from build123d import *

# Parameters (mm, degrees)
F1_DEPTH = 4.5
F2_DEPTH = 4.501
F3_DEPTH = 1
F4_R     = 2


# Not quite as in the source:
# - a feature names something its author has since deleted; it is built from what else it names


with BuildPart() as f1:
    # F0 (on Front) → F1 (new body)
    with BuildSketch(Plane.XZ):
        Polygon((25, 12.5), (-25, 12.5), (-25, 4), (-25, -4), (-25, -12.5), (25, -12.5), (25, -4), (25, 4), align=None)
        Polygon((-23.25, 7.75), (-23.25, 10.75), (-20.25, 10.75), (20.25, 10.75), (23.25, 10.75), (23.25, 7.75), (23.25, -7.75), (23.25, -10.75), (20.25, -10.75), (-20.25, -10.75), (-23.25, -10.75), (-23.25, -7.75), align=None, mode=Mode.SUBTRACT)
        Polygon((-20.25, 10.75), (-23.25, 10.75), (-23.25, 7.75), align=None)
        Polygon((23.25, 10.75), (20.25, 10.75), (23.25, 7.75), align=None)
        with BuildLine():
            Line((-25, -4), (-25, 4))
            Line((-25, 4), (-29.5, 4))
            ThreePointArc((-29.5, 4), (-33.5, 0), (-29.5, -4))
            Line((-29.5, -4), (-25, -4))
        make_face()
        with BuildLine():
            Line((-28.5, -1.8), (-29.5, -1.8))
            ThreePointArc((-29.5, -1.8), (-31.3, 0), (-29.5, 1.8))
            Line((-29.5, 1.8), (-28.5, 1.8))
            ThreePointArc((-28.5, 1.8), (-26.7, 0), (-28.5, -1.8))
        make_face(mode=Mode.SUBTRACT)
        with BuildLine():
            Line((29.5, 4), (25, 4))
            Line((25, 4), (25, -4))
            Line((25, -4), (29.5, -4))
            ThreePointArc((29.5, -4), (33.5, 0), (29.5, 4))
        make_face()
        with BuildLine():
            ThreePointArc((29.5, 1.8), (31.3, 0), (29.5, -1.8))
            Line((29.5, -1.8), (28.5, -1.8))
            ThreePointArc((28.5, -1.8), (26.7, 0), (28.5, 1.8))
            Line((28.5, 1.8), (29.5, 1.8))
        make_face(mode=Mode.SUBTRACT)
    extrude(amount=F1_DEPTH)

    # F0 (on Front) → F2 (cut, through all)
    with BuildSketch(Plane.XZ):
        Polygon((-20.25, 10.75), (-23.25, 10.75), (-23.25, 7.75), align=None)
        Polygon((20.25, 10.75), (-20.25, 10.75), (-23.25, 7.75), (-23.25, -7.75), (-20.25, -10.75), (20.25, -10.75), (23.25, -7.75), (23.25, 7.75), align=None)
        Polygon((23.25, 10.75), (20.25, 10.75), (23.25, 7.75), align=None)
    extrude(amount=F2_DEPTH, mode=Mode.SUBTRACT)

    # F0 (on Front) → F3 (join)
    with BuildSketch(Plane.XZ):
        Polygon((23.25, 10.75), (20.25, 10.75), (23.25, 7.75), align=None)
        Polygon((23.25, -10.75), (23.25, -7.75), (20.25, -10.75), align=None)
        Polygon((-20.25, 10.75), (-23.25, 10.75), (-23.25, 7.75), align=None)
        Polygon((-20.25, -10.75), (-23.25, -7.75), (-23.25, -10.75), align=None)
    extrude(amount=F3_DEPTH)

    # F4
    f4_edges = [f1.edges().sort_by_distance(p)[0] for p in [
        (-25, -2.25, -12.5),
        (25, -2.25, -12.5),
        (25, -2.25, 12.5),
        (-25, -2.25, 12.5),
    ]]
    fillet(f4_edges, radius=F4_R)


solid = f1.part
Source: CAD feature listing. Evaluate the final solid. Frame: model axes, mm. A direction names the side the tool comes from. Round coordinates to 2 decimals unless told otherwise and drop trailing zeros. Loops run counter-clockwise (first coordinate to the right, second up) from the corner with the lowest first, then second, coordinate; pieces in that order, holes last. Notation, with made-up numbers: M 23,60 L 41,60 A32 ccw 41,99 Z; hole C 50.25,-40 d1. An arc over 180 degrees is marked long. Return JSON: item names as keys, results as strings. Group by question number.
1. Reachability of faces 1 (the face through (-27, -2, 4)), 2 (the face through (-21.8, -0.5, 9.2)), 3 (the face through (22, -1, -10)) from +Z, -Z, +X, -X, +Y, -Y: full face, straight path, thin tool, end or side. Return the list, or none.
2. Mould query, pull axis Z, two halves, no side actions, for faces 4 (the face through (-21.7, -0.5, -9.3)), 5 (the face through (27, -2, 4)), 6 (the face through (24.4, -2.28, -11.93)), 7 (the face through (-25, -2, -7)). Classes: released by +Z, released by -Z, zero draft, split by the parting line, or undercut.
3. Section query A-A on x = -9. Output: boundary loops of the cut face in (y, z), and give its area (4 significant figures).
4. Section query C-C on y = -1.85. Output: boundary loops of the cut face in (x, z), and give its area (3 significant figures).
5. Section query B-B on z = 6.5. Output: boundary loops of the cut face in (x, y), and give its area (4 significant figures).
6. Material intervals for line 1 along Z through (x, y) = (-9.5, -3); line 2 along X through (y, z) = (-4.05, -4.25); line 3 along X through (y, z) = (-0.8, -8), sorted ascending. Write a range as from..to.
7. Pin query (flat end, axial travel): pin 1 (2 mm diameter, centred on x = 27, y = -1.5, fed in from +Z); pin 2 (2 mm diameter, centred on y = -1.5, z = -7, fed in from -X); pin 3 (1.5 mm diameter, centred on x = 22, z = -9, fed in from -Y). Return the tip coordinate at first contact, or that it passes through.
Checks:
{
 "1": {"face 1": "+Z, -X, +Y, -Y", "face 2": "+Y, -Y", "face 3": "-Y"},
 "2": {"face 4": "undercut", "face 5": "released by +Z", "face 6": "released by -Z", "face 7": "zero draft"},
 "3": {"outline": "M -4.5,-12.5 L 0,-12.5 L 0,-10.75 L -4.5,-10.75 Z; M -4.5,10.75 L 0,10.75 L 0,12.5 L -4.5,12.5 Z", "area": "15.75 mm²"},
 "4": {"outline": "M -29.5,-4 L -25,-4 L -25,-10.5 A2 ccw -23,-12.5 L 23,-12.5 A2 ccw 25,-10.5 L 25,-4 L 29.5,-4 A4 ccw 29.5,4 L 25,4 L 25,10.5 A2 ccw 23,12.5 L -23,12.5 A2 ccw -25,10.5 L -25,4 L -29.5,4 A4 ccw Z; hole M -29.5,-1.8 L -28.5,-1.8 A1.8 ccw -28.5,1.8 L -29.5,1.8 A1.8 ccw Z; hole M -23.25,-10.75 L 23.25,-10.75 L 23.25,10.75 L -23.25,10.75 Z; hole M 28.5,-1.8 L 29.5,-1.8 A1.8 ccw 29.5,1.8 L 28.5,1.8 A1.8 ccw Z", "area": "342 mm²"},
 "5": {"outline": "M -25,-4.5 L -23.25,-4.5 L -23.25,0 L -25,0 Z; M 23.25,-4.5 L 25,-4.5 L 25,0 L 23.25,0 Z", "area": "15.75 mm²"},
 "6": {"line 1": "z = -12.5..-10.75, 10.75..12.5", "line 2": "x = -25..-23.25, 23.25..25", "line 3": "x = -25..-23, 23..25"},
 "7": {"pin 1": "stops at z = 4", "pin 2": "stops at x = -25", "pin 3": "stops at y = -1"}
}
